Design review of the part built by this model. Coordinates are the model's own, in mm. A direction names the side the tool comes from. Give positions to 0.01 mm unless a question says otherwise; leave off trailing zeros. Write each loop counter-clockwise with the first axis right and the second up, starting at its lowest first coordinate (ties: lowest second). Pieces come first, ordered by that corner, then holes. Notation, with made-up numbers: M 53.5,48.5 L 107.5,48.5 A15 cw 107.5,56.5 Z; hole C 71,54.5 d9. An arc over 180 degrees is marked long. Answer in a Markdown table with one row per item.
```python
from build123d import *

# Parameters (mm, degrees)
BOSS_EXTRUDE1_DEPTH   = 80
CUT_EXTRUDE1_DEPTH    = 40
M4X0_7_TAPPED_HOLE1_D = 3.3


with BuildPart() as part:
    # Sketch1 → Boss-Extrude1 (new body)
    with BuildSketch(Plane.XY):
        Polygon((-4, 0), (4, 0), (19, 15), (19, 18), (-19, 18), (-19, 15), align=None)
    extrude(amount=BOSS_EXTRUDE1_DEPTH)

    # Sketch2 → Cut-Extrude1 (cut)
    with BuildSketch(Plane(origin=(0, 18, 0), x_dir=(1, 0, 0), z_dir=(0, 1, 0))):
        with BuildLine():
            Line((-10.25, -20), (-10.25, -60))
            ThreePointArc((-10.25, -60), (-12, -61.75), (-13.75, -60))
            Line((-13.75, -60), (-13.75, -20))
            ThreePointArc((-13.75, -20), (-12, -18.25), (-10.25, -20))
        make_face()
        with BuildLine():
            Line((13.75, -20), (13.75, -60))
            ThreePointArc((13.75, -60), (12, -61.75), (10.25, -60))
            Line((10.25, -60), (10.25, -20))
            ThreePointArc((10.25, -20), (12, -18.25), (13.75, -20))
        make_face()
    extrude(amount=-CUT_EXTRUDE1_DEPTH, mode=Mode.SUBTRACT)

    # M4x0.7 Tapped Hole1 (through all)
    with Locations(Plane(origin=(0, 18, 0), x_dir=(1, 0, 0), z_dir=(0, 1, 0))):
        with Locations((9.00246861, -10), (-15.99753139, -10)):
            Hole(M4X0_7_TAPPED_HOLE1_D / 2)


solid = part.part
```
1) To check wall thickness, follow probe 1 along X at (y, z) = (17.25, 32); probe 2 along X at (y, z) = (16, 10); probe 3 along X at (y, z) = (9.75, 10). State the ranges of each line that lie inside material, in increasing order. Write a range as [from, to].
Geometry says:
| item | result |
|---|---|
| probe 1 | [-19, -13.75], [-10.25, 10.25], [13.75, 19] |
| probe 2 | [-19, -17.65], [-14.35, 7.35], [10.65, 19] |
| probe 3 | [-13.75, 7.35], [10.65, 13.75] |
2) The part is to be moulded in two halves that separate along X. For faces 3 (the face through (13.75, 14, 40)), 4 (the face through (11.96, 13.51, 18.25)), 5 (the face through (-10, 6, 39)), 6 (the face through (0, 11, 80)), say which applies: released by +X, released by -X, zero draft, split by the parting line, or undercut.
Geometry says:
| item | result |
|---|---|
| face 3 | undercut |
| face 4 | undercut |
| face 5 | released by -X |
| face 6 | zero draft |
3) Add section B-B (z = 19). Write out the cut boundary in (x, y), and give its area (3 significant figures).
Geometry says:
| item | result |
|---|---|
| outline | M -19,15 L -13.44,9.44 L -13.44,18 L -19,18 Z; M -10.56,6.56 L -4,0 L 4,0 L 10.56,6.56 L 10.56,18 L -10.56,18 Z; M 13.44,9.44 L 19,15 L 19,18 L 13.44,18 Z |
| area | 402 mm^2 |
4) Add section C-C (y = 7.25). Write out the cut boundary in (x, z), and give its area (3 significant figures).
Geometry says:
| item | result |
|---|---|
| outline | M -11.25,0 L 11.25,0 L 11.25,18.42 A1.75 cw 10.25,20 L 10.25,60 A1.75 cw 11.25,61.58 L 11.25,80 L -11.25,80 L -11.25,61.58 A1.75 cw -10.25,60 L -10.25,20 A1.75 cw -11.25,18.42 Z; hole C 9,10 d3.3 |
| area | 1,710 mm^2 |
5) Insertion check: P1, Ø1, axis at y = 2, z = 48, coming from the -X side; P2, Ø3, axis at x = -0.5, z = 53.5, coming from the -Y side; P3, Ø4, axis at x = -7.5, z = 24, coming from the -Y side; P4, Ø6, axis at y = 10, z = 47, coming from the +X side. Each pin has a flat end and moves straight along its axis. Give the tip position at first contact, or say it passes through.
Geometry says:
| item | result |
|---|---|
| P1 | x = -6.5 |
| P2 | y = 0 |
| P3 | y = 1.5 |
| P4 | x = 17 |
6) For faces 1 (the face through (12.04, 13.51, 61.75)), 2 (the face through (0, 0, 39)), list the 3-axis set-ups (+Z, -Z, +X, -X, +Y, -Y) from which the entire face can be reached by the end or side of a thin tool; tool diameter is ignored.
Geometry says:
| item | result |
|---|---|
| face 1 | +Y, -Y |
| face 2 | +Z, -Z, +X, -X, -Y |
7) Add section D-D (z = 30). Write out the cut boundary in (x, y), and give its area (3 significant figures).
Geometry says:
| item | result |
|---|---|
| outline | M -19,15 L -13.75,9.75 L -13.75,18 L -19,18 Z; M -10.25,6.25 L -4,0 L 4,0 L 10.25,6.25 L 10.25,18 L -10.25,18 Z; M 13.75,9.75 L 19,15 L 19,18 L 13.75,18 Z |
| area | 389 mm^2 |
8) Add section A-A (x = -12). Write out the cut boundary in (y, z), and give its area (3 significant figures).
Geometry says:
| item | result |
|---|---|
| outline | M 8,0 L 18,0 L 18,18.25 L 8,18.25 Z; M 8,61.75 L 18,61.75 L 18,80 L 8,80 Z |
| area | 365 mm^2 |
